Geometry: see drawing. Coordinates: mm, zero at the bounding-box minimum. A direction names the side the tool comes from. Coordinates: 2 decimals unless noted, no trailing zeros. Order: outer loops, then holes, each group sorted by start corner. A loop starts at its lowest first (then second) coordinate and runs counter-clockwise, first axis right, second up. Notation, with made-up numbers: (-38, -3.75) - (18, -3.75) arc R23 cw to (18, 24.25) - close; hole circle Ø10 at (80.25, 25). An arc over 180 degrees is marked (long way). Use a Markdown table: item, result. Add a question column.
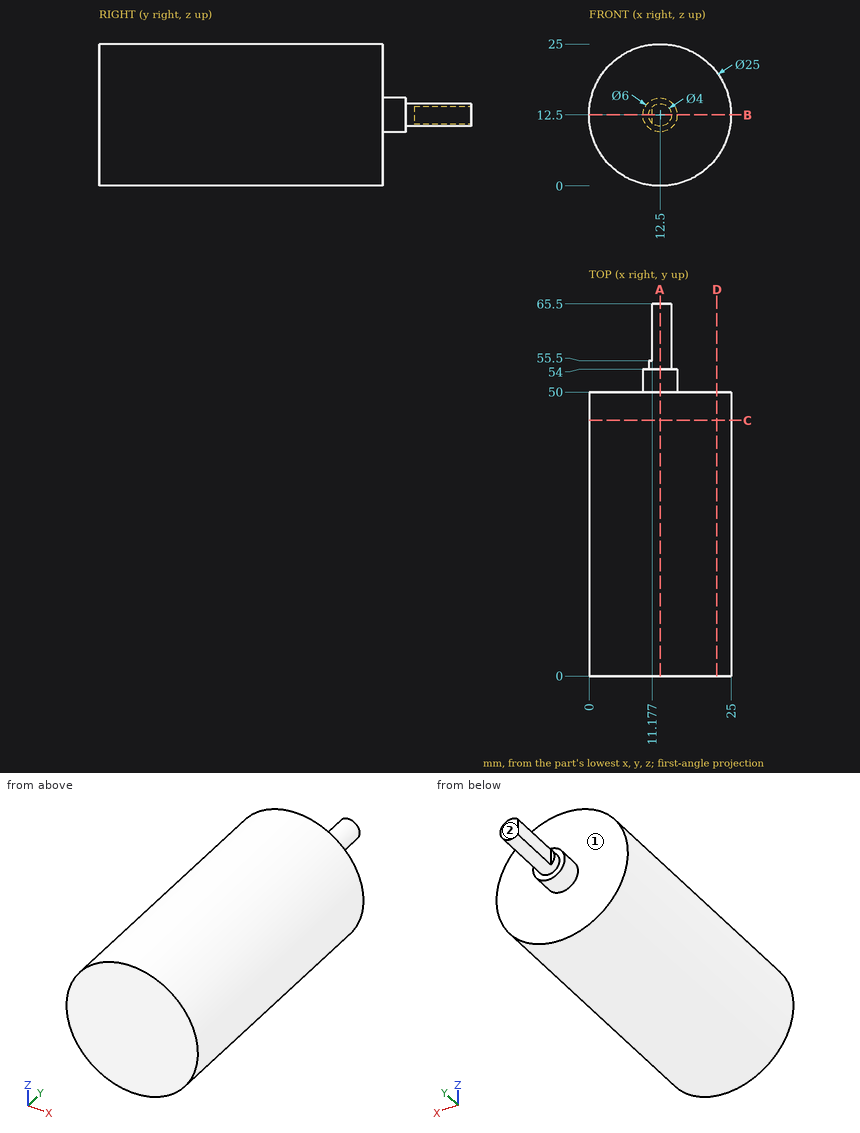
1) Cut plane B-B (z = 12.5). Return the cut outline in (x, y), and give its area (3 significant figures).
2) Cut plane A-A (x = 12.5). Return the cut outline in (y, z), and give its area (3 significant figures).
3) Reachability of the marked faces 1 and 2 from +Z, -Z, +X, -X, +Y, -Y: full face, straight path, thin tool, end or side. Return the list, or none.
4) Cut plane C-C (y = 45). Return the cut outline in (x, z), and give its area (3 significant figures).
5) Material intervals for L1, parallel to Z at x = 13, y = 27; L2, parallel to Y at x = 5.75, z = 18.75; L3, parallel to X at y = 24.5, z = 12.75, sorted ascending.
6) Cut plane D-D (x = 22.5). Return the cut outline in (y, z).
7) Contact query for flat-ended pins moving along their axis: P1, Ø6, axis at x = 6.5, y = 7.5, coming from the -Z side; P2, Ø3.5, axis at y = 62.5, z = 13, coming from the -X side; P3, Ø3, axis at x = 2.5, y = 21.5, coming from the -Z side (1 decimal). Output: stop coordinate, or through.
Computed:
| question | item | result |
|---|---|---|
| 1 | outline | (0, 0) - (25, 0) - (25, 50) - (15.5, 50) - (15.5, 54) - (14.5, 54) - (14.5, 65.5) - (11.18, 65.5) - (11.18, 55.5) - (10.5, 55.5) - (10.5, 54) - (9.5, 54) - (9.5, 50) - (0, 50) - close |
| 1 | area | 1,310 mm2 |
| 2 | outline | (0, 0) - (50, 0) - (50, 9.5) - (54, 9.5) - (54, 10.5) - (65.5, 10.5) - (65.5, 14.5) - (54, 14.5) - (54, 15.5) - (50, 15.5) - (50, 25) - (0, 25) - close |
| 2 | area | 1,320 mm2 |
| 3 | face 1 | +Y |
| 3 | face 2 | +Z, -Z, +X, -X, +Y |
| 4 | outline | circle Ø25 at (12.5, 12.5) |
| 4 | area | 491 mm2 |
| 5 | L1 | z = 0.01 to 24.99 |
| 5 | L2 | y = 0 to 50 |
| 5 | L3 | x = 0 to 25 |
| 6 | outline | (0, 5) - (50, 5) - (50, 20) - (0, 20) - close |
| 7 | P1 | stops at z = 0.37 |
| 7 | P2 | stops at x = 11.18 |
| 7 | P3 | stops at z = 3.3 |
